Could you check a few things on this model? Use its own coordinates, in mm. Face numbers are marked on the shaded views. A direction names the side the tool comes from. Coordinates: 2 decimals unless noted, no trailing zeros. Loops run counter-clockwise (first coordinate to the right, second up) from the corner with the lowest first, then second, coordinate; pieces in that order, holes last.
1) Imagine slicing it at C-C on y = 20. Please give me the cut outline in (x, z), plus the area to 3 significant figures.
2) Imagine slicing it at B-B on z = -79. Please give me the cut outline in (x, y), plus the area to 3 significant figures.
3) If I drill on line 1 along Z through (x, y) = (20, -1); line 2 along X through (y, z) = (-5.5, -145); line 3 along Y through (x, z) = (27, -58), over which ranges is the centre line in solid material (lowest first)?
4) Imagine slicing it at D-D on x = 38. Please give me the cut outline in (y, z).
5) Will these pins go through, and if not, where does the flat tip stop? P1, Ø10, axis at y = 6, z = -90, coming from the +X side; P2, Ø4, axis at x = 65.5, y = 20.5, coming from the -Z side; P3, Ø5, axis at y = -5, z = -118.5, coming from the +X side.
6) Thinking about a two-plate mould opening in X: for the marked faces 1, 2 and 3, which applies, released by +X, released by -X, zero draft, split by the parting line, or undercut?
7) Imagine slicing it at A-A on y = -7. Please give me the cut outline in (x, z).
8) For the marked faces 4, 5 and 6, which set-ups out of +Z, -Z, +X, -X, +Y, -Y let a thin tool reach every point of the face, with its end or its side?
```python
from build123d import *

# Parameters (mm, degrees)
F0_W     = 10
F0_H     = 10
F1_DEPTH = 25
F2_DEPTH = 10
F3_R     = 10
F5_DEPTH = 10
F7_D     = 5
F7_DEPTH = 11.19
F7_TIP   = 1.5021515476


with BuildPart() as f1:
    # F0 (on Front) → F1 (new body)
    with BuildSketch(Plane.XZ):
        with BuildLine():
            Line((15, -40), (0, -40))
            Line((0, -40), (0, -160))
            Line((0, -160), (40, -160))
            Line((40, -160), (40, -85))
            Line((40, -85), (40, -75))
            Line((40, -75), (40, -55))
            Line((40, -55), (40, -45))
            Line((40, -45), (40, -40))
            Line((40, -40), (25, -40))
            ThreePointArc((25, -40), (28.5355339059, -41.4644660941), (30, -45))
            Line((30, -45), (30, -55))
            ThreePointArc((30, -55), (28.5355339059, -58.5355339059), (25, -60))
            Line((25, -60), (15, -60))
            ThreePointArc((15, -60), (11.4644660941, -58.5355339059), (10, -55))
            Line((10, -55), (10, -45))
            ThreePointArc((10, -45), (11.4644660941, -41.4644660941), (15, -40))
        make_face()
        with BuildLine():
            Line((25, -90), (15, -90))
            ThreePointArc((15, -90), (11.4644660941, -88.5355339059), (10, -85))
            Line((10, -85), (10, -75))
            ThreePointArc((10, -75), (11.4644660941, -71.4644660941), (15, -70))
            Line((15, -70), (25, -70))
            ThreePointArc((25, -70), (28.5355339059, -71.4644660941), (30, -75))
            Line((30, -75), (30, -85))
            ThreePointArc((30, -85), (28.5355339059, -88.5355339059), (25, -90))
        make_face(mode=Mode.SUBTRACT)
        Polygon((40, 0), (10, 0), (10, -10), (0, -10), (0, -40), (15, -40), (25, -40), (40, -40), (40, -25), (40, -15), align=None)
        with BuildLine():
            ThreePointArc((10, -15), (11.4644660941, -11.4644660941), (15, -10))
            Line((15, -10), (25, -10))
            ThreePointArc((25, -10), (28.5355339059, -11.4644660941), (30, -15))
            Line((30, -15), (30, -25))
            ThreePointArc((30, -25), (28.5355339059, -28.5355339059), (25, -30))
            Line((25, -30), (15, -30))
            ThreePointArc((15, -30), (11.4644660941, -28.5355339059), (10, -25))
            Line((10, -25), (10, -15))
        make_face(mode=Mode.SUBTRACT)
        with Locations((5, -5)):
            Rectangle(F0_W, F0_H)
        with BuildLine():
            Line((130, 0), (40, 0))
            Line((40, 0), (40, -15))
            ThreePointArc((40, -15), (41.4644660941, -11.4644660941), (45, -10))
            Line((45, -10), (55, -10))
            ThreePointArc((55, -10), (58.5355339059, -11.4644660941), (60, -15))
            Line((60, -15), (60, -25))
            ThreePointArc((60, -25), (58.5355339059, -28.5355339059), (55, -30))
            Line((55, -30), (45, -30))
            ThreePointArc((45, -30), (41.4644660941, -28.5355339059), (40, -25))
            Line((40, -25), (40, -40))
            Line((40, -40), (45, -40))
            Line((45, -40), (55, -40))
            Line((55, -40), (75, -40))
            Line((75, -40), (85, -40))
            Line((85, -40), (105, -40))
            Line((105, -40), (115, -40))
            Line((115, -40), (130, -40))
            Line((130, -40), (130, 0))
        make_face()
        with BuildLine():
            Line((85, -30), (75, -30))
            ThreePointArc((75, -30), (71.4644660941, -28.5355339059), (70, -25))
            Line((70, -25), (70, -15))
            ThreePointArc((70, -15), (71.4644660941, -11.4644660941), (75, -10))
            Line((75, -10), (85, -10))
            ThreePointArc((85, -10), (88.5355339059, -11.4644660941), (90, -15))
            Line((90, -15), (90, -25))
            ThreePointArc((90, -25), (88.5355339059, -28.5355339059), (85, -30))
        make_face(mode=Mode.SUBTRACT)
        with BuildLine():
            Line((115, -30), (105, -30))
            ThreePointArc((105, -30), (101.4644660941, -28.5355339059), (100, -25))
            Line((100, -25), (100, -15))
            ThreePointArc((100, -15), (101.4644660941, -11.4644660941), (105, -10))
            Line((105, -10), (115, -10))
            ThreePointArc((115, -10), (118.5355339059, -11.4644660941), (120, -15))
            Line((120, -15), (120, -25))
            ThreePointArc((120, -25), (118.5355339059, -28.5355339059), (115, -30))
        make_face(mode=Mode.SUBTRACT)
        with BuildLine():
            ThreePointArc((10, -85), (11.4644660941, -88.5355339059), (15, -90))
            Line((15, -90), (25, -90))
            ThreePointArc((25, -90), (28.5355339059, -88.5355339059), (30, -85))
            Line((30, -85), (30, -75))
            ThreePointArc((30, -75), (28.5355339059, -71.4644660941), (25, -70))
            Line((25, -70), (15, -70))
            ThreePointArc((15, -70), (11.4644660941, -71.4644660941), (10, -75))
            Line((10, -75), (10, -85))
        make_face()
        with BuildLine():
            Line((25, -40), (15, -40))
            ThreePointArc((15, -40), (11.4644660941, -41.4644660941), (10, -45))
            Line((10, -45), (10, -55))
            ThreePointArc((10, -55), (11.4644660941, -58.5355339059), (15, -60))
            Line((15, -60), (25, -60))
            ThreePointArc((25, -60), (28.5355339059, -58.5355339059), (30, -55))
            Line((30, -55), (30, -45))
            ThreePointArc((30, -45), (28.5355339059, -41.4644660941), (25, -40))
        make_face()
        with BuildLine():
            Line((25, -10), (15, -10))
            ThreePointArc((15, -10), (11.4644660941, -11.4644660941), (10, -15))
            Line((10, -15), (10, -25))
            ThreePointArc((10, -25), (11.4644660941, -28.5355339059), (15, -30))
            Line((15, -30), (25, -30))
            ThreePointArc((25, -30), (28.5355339059, -28.5355339059), (30, -25))
            Line((30, -25), (30, -15))
            ThreePointArc((30, -15), (28.5355339059, -11.4644660941), (25, -10))
        make_face()
        with BuildLine():
            ThreePointArc((45, -10), (41.4644660941, -11.4644660941), (40, -15))
            Line((40, -15), (40, -25))
            ThreePointArc((40, -25), (41.4644660941, -28.5355339059), (45, -30))
            Line((45, -30), (55, -30))
            ThreePointArc((55, -30), (58.5355339059, -28.5355339059), (60, -25))
            Line((60, -25), (60, -15))
            ThreePointArc((60, -15), (58.5355339059, -11.4644660941), (55, -10))
            Line((55, -10), (45, -10))
        make_face()
        with BuildLine():
            ThreePointArc((70, -25), (71.4644660941, -28.5355339059), (75, -30))
            Line((75, -30), (85, -30))
            ThreePointArc((85, -30), (88.5355339059, -28.5355339059), (90, -25))
            Line((90, -25), (90, -15))
            ThreePointArc((90, -15), (88.5355339059, -11.4644660941), (85, -10))
            Line((85, -10), (75, -10))
            ThreePointArc((75, -10), (71.4644660941, -11.4644660941), (70, -15))
            Line((70, -15), (70, -25))
        make_face()
        with BuildLine():
            ThreePointArc((100, -25), (101.4644660941, -28.5355339059), (105, -30))
            Line((105, -30), (115, -30))
            ThreePointArc((115, -30), (118.5355339059, -28.5355339059), (120, -25))
            Line((120, -25), (120, -15))
            ThreePointArc((120, -15), (118.5355339059, -11.4644660941), (115, -10))
            Line((115, -10), (105, -10))
            ThreePointArc((105, -10), (101.4644660941, -11.4644660941), (100, -15))
            Line((100, -15), (100, -25))
        make_face()
    extrude(amount=-F1_DEPTH)

    # F0 (on Front) → F2 (cut)
    with BuildSketch(Plane.XZ):
        with BuildLine():
            Line((25, -10), (15, -10))
            ThreePointArc((15, -10), (11.4644660941, -11.4644660941), (10, -15))
            Line((10, -15), (10, -25))
            ThreePointArc((10, -25), (11.4644660941, -28.5355339059), (15, -30))
            Line((15, -30), (25, -30))
            ThreePointArc((25, -30), (28.5355339059, -28.5355339059), (30, -25))
            Line((30, -25), (30, -15))
            ThreePointArc((30, -15), (28.5355339059, -11.4644660941), (25, -10))
        make_face()
        with BuildLine():
            ThreePointArc((45, -10), (41.4644660941, -11.4644660941), (40, -15))
            Line((40, -15), (40, -25))
            ThreePointArc((40, -25), (41.4644660941, -28.5355339059), (45, -30))
            Line((45, -30), (55, -30))
            ThreePointArc((55, -30), (58.5355339059, -28.5355339059), (60, -25))
            Line((60, -25), (60, -15))
            ThreePointArc((60, -15), (58.5355339059, -11.4644660941), (55, -10))
            Line((55, -10), (45, -10))
        make_face()
        with BuildLine():
            ThreePointArc((70, -25), (71.4644660941, -28.5355339059), (75, -30))
            Line((75, -30), (85, -30))
            ThreePointArc((85, -30), (88.5355339059, -28.5355339059), (90, -25))
            Line((90, -25), (90, -15))
            ThreePointArc((90, -15), (88.5355339059, -11.4644660941), (85, -10))
            Line((85, -10), (75, -10))
            ThreePointArc((75, -10), (71.4644660941, -11.4644660941), (70, -15))
            Line((70, -15), (70, -25))
        make_face()
        with BuildLine():
            ThreePointArc((100, -25), (101.4644660941, -28.5355339059), (105, -30))
            Line((105, -30), (115, -30))
            ThreePointArc((115, -30), (118.5355339059, -28.5355339059), (120, -25))
            Line((120, -25), (120, -15))
            ThreePointArc((120, -15), (118.5355339059, -11.4644660941), (115, -10))
            Line((115, -10), (105, -10))
            ThreePointArc((105, -10), (101.4644660941, -11.4644660941), (100, -15))
            Line((100, -15), (100, -25))
        make_face()
        with BuildLine():
            Line((25, -40), (15, -40))
            ThreePointArc((15, -40), (11.4644660941, -41.4644660941), (10, -45))
            Line((10, -45), (10, -55))
            ThreePointArc((10, -55), (11.4644660941, -58.5355339059), (15, -60))
            Line((15, -60), (25, -60))
            ThreePointArc((25, -60), (28.5355339059, -58.5355339059), (30, -55))
            Line((30, -55), (30, -45))
            ThreePointArc((30, -45), (28.5355339059, -41.4644660941), (25, -40))
        make_face()
        with BuildLine():
            ThreePointArc((10, -85), (11.4644660941, -88.5355339059), (15, -90))
            Line((15, -90), (25, -90))
            ThreePointArc((25, -90), (28.5355339059, -88.5355339059), (30, -85))
            Line((30, -85), (30, -75))
            ThreePointArc((30, -75), (28.5355339059, -71.4644660941), (25, -70))
            Line((25, -70), (15, -70))
            ThreePointArc((15, -70), (11.4644660941, -71.4644660941), (10, -75))
            Line((10, -75), (10, -85))
        make_face()
    extrude(amount=-F2_DEPTH, mode=Mode.SUBTRACT)

    # F3
    f3_edges = [f1.edges().sort_by_distance(p)[0] for p in [
        (0, 12.5, -160),
        (40, 12.5, -160),
        (40, 12.5, -40),
        (130, 12.5, -40),
        (130, 12.5, 0),
        (0, 12.5, 0),
    ]]
    fillet(f3_edges, radius=F3_R)

    # F4 (on face) → F5 (join)
    with BuildSketch(Plane.XZ):
        with BuildLine():
            ThreePointArc((12.5, -145), (14.6966991411, -150.3033008589), (20, -152.5))
            ThreePointArc((20, -152.5), (25.3033008589, -150.3033008589), (27.5, -145))
            Line((27.5, -145), (27.5, -105))
            ThreePointArc((27.5, -105), (20, -97.5), (12.5, -105))
            Line((12.5, -105), (12.5, -145))
        make_face()
    extrude(amount=F5_DEPTH)

    # F7
    with Locations(Plane.XZ.offset(10)):
        with Locations((20, -105), (20, -145)):
            Hole(F7_D / 2, depth=F7_DEPTH)
            with Locations((0, 0, -(F7_DEPTH + F7_TIP / 2))):  # 118° drill point
                Cone(0, F7_D / 2, F7_TIP, mode=Mode.SUBTRACT)


solid = f1.part
```
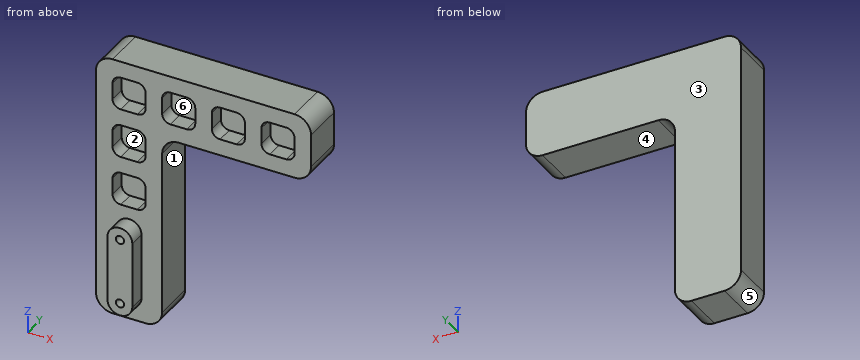
Filled in:
1. outline: (0, -150) arc R10 ccw to (10, -160) - (30, -160) arc R10 ccw to (40, -150) - (40, -50) arc R10 cw to (50, -40) - (120, -40) arc R10 ccw to (130, -30) - (130, -10) arc R10 ccw to (120, 0) - (10, 0) arc R10 ccw to (0, -10) - close
1. area: 9,910 mm2
2. outline: (0, 0) - (10, 0) - (10, 10) - (30, 10) - (30, 0) - (40, 0) - (40, 25) - (0, 25) - close
2. area: 800 mm2
3. line 1: z = -152.5 to -147.5, -142.5 to -107.5, -102.5 to -97.5
3. line 2: x = 12.5 to 17.5, 22.5 to 27.5
3. line 3: y = 10 to 25
4. outline: (0, -156) - (25, -156) - (25, 0) - (0, 0) - close
5. P1: stops at x = 40
5. P2: stops at z = -40
5. P3: stops at x = 27.5
6. face 1: released by +X
6. face 2: undercut
6. face 3: zero draft
7. outline: (12.5, -145) arc R7.5 ccw to (27.5, -145) - (27.5, -105) arc R7.5 ccw to (12.5, -105) - close; hole circle Ø5 at (20, -145); hole circle Ø5 at (20, -105)
8. face 4: -Z, +X, +Y, -Y
8. face 5: -Z, -X, +Y, -Y
8. face 6: -Y
